Here's how the part is built. I have some questions about the finished solid (model axes, mm). A direction names the side the tool comes from. Round coordinates to 2 decimals unless told otherwise and drop trailing zeros. Order: outer loops, then holes, each group sorted by start corner. A loop starts at its lowest first (then second) coordinate and runs counter-clockwise, first axis right, second up. Notation, with made-up numbers: (-27.75, 88.5) -> (20.25, 88.5) arc R22 cw to (20.25, 119.5) -> close; hole circle Ø7 at (-7, -23.5). An arc over 180 degrees is marked (long way). Use a Markdown table: item, result. Add a question column.
(1) I'm going to push flat-ended pins straight in: P1, Ø2, axis at x = -28, z = 10, coming from the +Y side; P2, Ø3, axis at x = -20.5, z = 14.5, coming from the -Y side; P3, Ø8, axis at y = -46.5, z = 12, coming from the -X side. Where does each tip first touch, or does it pass through?
(2) I want a section at B-B, the plane z = 18.75. Please give me the cut outline in (x, y), then the cut area to 3 significant figures.
(3) I want a section at D-D, the plane y = 22.5. Please give me the cut outline in (x, z).
(4) I want a section at A-A, the plane x = -6. Please give me the cut outline in (y, z), then the cut area to 3 significant figures.
(5) I want a section at C-C, the plane y = -10. Please give me the cut outline in (x, z) (3 decimals).
(6) On a 3-axis mill with a long thin cutter (end or side, diameter ignored), from which of +Z, -Z, +X, -X, +Y, -Y can I reach the whole of each face in a straight line? I mean faces 1 (the face through (-17, -3, 7.058)), 2 (the face through (0.649, -34.525, 11.104)). Say none if no direction works.
(7) If I drill on probe 1 along Y at (x, z) = (-41, 20.25); probe 2 along Y at (x, z) = (0, 13); probe 3 along X at (y, z) = (-37.5, 14.75), over which ranges is the centre line in solid material (lowest first)?
from build123d import *

# Parameters (mm, degrees)
F1_DEPTH = 6.35
F5_R     = 0.8255
F6_DEPTH = 76.2
F4_R     = 3.175
F7_DEPTH = 57.15


with BuildPart() as f1:
    # F0 (on Front) → F1 (new body)
    with BuildSketch(Plane.XZ):
        with BuildLine():
            Line((8.678272, 21.247713), (-42.121728, 21.247713))
            ThreePointArc((-42.121728, 21.247713), (-49.216529, 14.152912), (-42.121728, 7.058111))
            Line((-42.121728, 7.058111), (8.678272, 7.058111))
            Line((8.678272, 7.058111), (8.678272, 21.247713))
        make_face()
    extrude(amount=F1_DEPTH)

    # F5 (on face) → F6 (join)
    with BuildSketch(Plane.XZ.offset(6.35)):
        with Locations((-42.576857, 14.333389)):
            Circle(F5_R)
    extrude(amount=-F6_DEPTH)

    # F4 (on face) → F7 (join)
    with BuildSketch(Plane.XZ.offset(6.35)):
        with Locations((1.337771, 14.203422)):
            Circle(F4_R)
    extrude(amount=F7_DEPTH)


solid = f1.part
Taken from the geometry:
| question | item | result |
|---|---|---|
| 1 | P1 | stops at y = 0 |
| 1 | P2 | stops at y = -6.35 |
| 1 | P3 | stops at x = -1.84 |
| 2 | outline | (-47.53, -6.35) -> (8.68, -6.35) -> (8.68, 0) -> (-47.53, 0) -> close |
| 2 | area | 357 mm2 |
| 3 | outline | circle Ø1.65 at (-42.58, 14.33) |
| 4 | outline | (-6.35, 7.06) -> (0, 7.06) -> (0, 21.25) -> (-6.35, 21.25) -> close |
| 4 | area | 90.1 mm2 |
| 5 | outline | circle Ø6.35 at (1.338, 14.203) |
| 6 | face 1 | -Z, +X, -X, +Y, -Y |
| 6 | face 2 | -Y |
| 7 | probe 1 | y = -6.35 to 0 |
| 7 | probe 2 | y = -63.5 to 0 |
| 7 | probe 3 | x = -1.79 to 4.47 |
